Autodesk Inventor part; units mm, degrees
ref_plane "YZ Plane" through (0, 0, 0) normal (1, 0, 0) x (0, 1, 0)
ref_plane "XZ Plane" through (0, 0, 0) normal (0, 1, 0) x (-1, 0, 0)
ref_plane "XY Plane" through (0, 0, 0) normal (0, 0, 1) x (1, 0, 0)
sketch "Sketch6" plane through (0, 0, 0) normal (0, 1, 0) x (-1, 0, 0)
  circle A0 centre (0, 0) radius 8.75
  circle A1 centre (0, 0) radius 4.5
  dimension "d18" = 17.5
  dimension "d35" = 9
extrude "Extrusion5" add sketch "Sketch6" along normal blind 36
sketch "Sketch10" plane through (0, 0, 0) normal (0, -1, 0) x (1, 0, 0)
  circle A0 centre (0, 0) radius 6.35
  dimension "d32" = 12.7
extrude "Extrusion8" cut sketch "Sketch10" against normal blind 32.6
sketch "Sketch11" plane through (0, 32.6, 0) normal (0, -1, 0) x (1, 0, 0)
  arc A0 (-4.2968, -4.4) -> (4.2968, -4.4) centre (0, 0) ccw
  line L0 (-4.2968, 4.4) -> (-16.8146, 2.7257)
  arc A1 (-16.8146, 2.7257) -> (-16.8146, -2.7257) centre (-16.45, 0) ccw
  line L1 (-16.8146, -2.7257) -> (-4.2968, -4.4)
  line L2 (4.2968, -4.4) -> (16.8146, -2.7257)
  arc A2 (16.8146, -2.7257) -> (16.8146, 2.7257) centre (16.45, 0) ccw
  line L3 (16.8146, 2.7257) -> (4.2968, 4.4)
  line L4 (-4.2968, -4.4) -> (4.2968, -4.4) construction
  line L5 (-4.2968, 4.4) -> (4.2968, 4.4) construction
  line L6 (-19.2, 0) -> (19.2, 0) construction
  arc A3 (-6.15, 0) -> (-4.2968, -4.4) centre (0, 0) ccw construction
  arc A4 (-4.2968, 4.4) -> (-6.15, 0) centre (0, 0) ccw construction
  arc A5 (4.2968, 4.4) -> (-4.2968, 4.4) centre (0, 0) ccw
  arc A6 (6.15, 0) -> (4.2968, 4.4) centre (0, 0) ccw construction
  arc A7 (4.2968, -4.4) -> (6.15, 0) centre (0, 0) ccw construction
  line L7 (-4.3428, -4.4947) -> (-16.8278, -2.8248)
  arc A8 (-16.8278, 2.8248) -> (-16.8278, -2.8248) centre (-16.45, 0) ccw
  line L8 (-16.8278, 2.8248) -> (-4.3428, 4.4947)
  arc A9 (4.3428, 4.4947) -> (-4.3428, 4.4947) centre (0, 0) ccw
  line L9 (4.3428, 4.4947) -> (16.8278, 2.8248)
  arc A10 (16.8278, -2.8248) -> (16.8278, 2.8248) centre (16.45, 0) ccw
  line L10 (16.8278, -2.8248) -> (4.3428, -4.4947)
  arc A11 (-4.3428, -4.4947) -> (4.3428, -4.4947) centre (0, 0) ccw
  point P0 (0, 0)
  point P1 (0, 0)
  dimension "d36" = 12.3
  dimension "d37" = 8.8
  dimension "d38" = 38.4
  dimension "d39" = 2.75
  dimension "d40" = 0.1
extrude "Extrusion9" cut sketch "Sketch11" along normal blind 29.2 contours L1 A1 L0 A5 L3 A2 L2 A0 | L7 A8 L8 A9 L9 A10 L10 A11
properties part number "attachmentcustom" material "PET Plastic"
The model under review builds one solid part; all positions refer to its coordinate system, in mm. A direction names the side the tool comes from. Round coordinates to 2 decimals unless told otherwise and drop trailing zeros. Loops run counter-clockwise (first coordinate to the right, second up) from the corner with the lowest first, then second, coordinate; pieces in that order, holes last. Notation, with made-up numbers: M 84.5,38 L 140.5,38 A11 ccw 140.5,58 Z; hole C 55.5,-39.75 d9. An arc over 180 degrees is marked long. Answer as a JSON object with one key per item and string values.
(1) Take a section at B-B on z = 0. Give the boundary of the cut face in (x, y), and give its area (3 significant figures).
Resolved:
{"outline": "M -8.75,0 L -6.35,0 L -6.35,3.4 L -8.75,3.4 Z; M -8.75,32.6 L -4.5,32.6 L -4.5,36 L -8.75,36 Z; M 4.5,32.6 L 8.75,32.6 L 8.75,36 L 4.5,36 Z; M 6.35,0 L 8.75,0 L 8.75,3.4 L 6.35,3.4 Z", "area": "45.2 mm²"}
(2) Tool access review of faces 4 (the cylindrical face through (6.944, 17.748, 5.324)), 5 (the flat face through (6.11, 18.2, 4.26)), 6 (the cylindrical face through (3.414, 16.072, 5.354)): name each direction out of +Z, -Z, +X, -X, +Y, -Y from which nothing blocks a thin tool from reaching the whole face with its end or side.
Resolved:
{"face 4": "+Y, -Y", "face 5": "none", "face 6": "-Y"}
(3) Take a section at A-A on y = 27. Give the boundary of the cut face in (x, z), and give its area (3 significant figures).
Resolved:
{"outline": "M -7.76,-4.04 A8.75 ccw 7.76,-4.04 L 4.51,-4.47 A6.35 cw -4.51,-4.47 Z; M -7.76,4.04 L -4.51,4.47 A6.35 cw 4.51,4.47 L 7.76,4.04 A8.75 ccw Z", "area": "70.4 mm²"}
(4) Take a section at C-C on x = 0. Give the boundary of the cut face in (y, z).
Resolved:
{"outline": "M 0,-8.75 L 36,-8.75 L 36,-4.5 L 32.6,-4.5 L 32.6,-6.35 L 0,-6.35 Z; M 0,6.35 L 32.6,6.35 L 32.6,4.5 L 36,4.5 L 36,8.75 L 0,8.75 Z"}
(5) Take a section at D-D on x = -7. Give the boundary of the cut face in (y, z), and give its area (3 significant figures).
Resolved:
{"outline": "M 0,-5.25 L 36,-5.25 L 36,5.25 L 0,5.25 Z; hole M 3.4,-4.14 L 32.6,-4.14 L 32.6,4.14 L 3.4,4.14 Z", "area": "136 mm²"}
(6) To check wall thickness, follow line 1 along Z through (x, y) = (0, 35); line 2 along Z through (x, y) = (0, 16); line 3 along Y through (x, z) = (-7.5, 2.5). State the ranges of each line that lie inside material, in increasing order.
Resolved:
{"line 1": "-8.75 to -4.5, 4.5 to 8.75", "line 2": "-8.75 to -6.35, 6.35 to 8.75", "line 3": "0 to 3.4, 32.6 to 36"}
(7) Clearance check with flat-ended pins moving along their axes: P1, Ø8, axis at x = 0, z = 0, coming from the +Y side; P2, Ø6, axis at x = 7, z = 5, coming from the -Y side; P3, Ø6, axis at x = -4, y = 30.5, coming from the -Z side; P4, Ø1, axis at x = 3, z = 4, coming from the -Y side. State where each tip first meets the part, or that it passes through.
Resolved:
{"P1": "through", "P2": "y = 0", "P3": "z = -8.69", "P4": "y = 32.6"}
(8) Draft analysis for pull direction Y (two halves, no side actions). For faces 1 (the flat face through (-4, 36, -4)), 2 (the flat face through (-4, 32.6, -3)), 3 (the cylindrical face through (0.59, 34.28, -4.46)), state which applies: released by +Y, released by -Y, zero draft, split by the parting line, or undercut.
Resolved:
{"face 1": "released by +Y", "face 2": "undercut", "face 3": "zero draft"}
